```python
from build123d import *

# Parameters (mm, degrees)
BOSS_EXTRUDE2_DEPTH = 50.8
CUT_EXTRUDE2_START  = -10.16
SKETCH2_R           = 6.35
CUT_EXTRUDE2_DEPTH  = 19.997379


with BuildPart() as part:
    # Sketch1 → Boss-Extrude2 (new body)
    with BuildSketch(Plane.XY):
        with BuildLine():
            Line((-2.54, 7.184204897), (-2.54, 9.837377699))
            ThreePointArc((-2.54, 9.837377699), (-6.221703947, -8.032185257), (10.16, 0))
            ThreePointArc((10.16, 0), (8.032185257, 6.221703947), (2.54, 9.837377699))
            Line((2.54, 9.837377699), (2.54, 7.184204897))
            ThreePointArc((2.54, 7.184204897), (6.221703947, 4.399409051), (7.62, 0))
            ThreePointArc((7.62, 0), (-4.399409051, -6.221703947), (-2.54, 7.184204897))
        make_face()
    extrude(amount=BOSS_EXTRUDE2_DEPTH)

    # Sketch2 → Cut-Extrude2 (cut)
    with BuildSketch(Plane(origin=(0, 0, 0), x_dir=(1, 0, 0), z_dir=(0, 1, 0)).offset(CUT_EXTRUDE2_START)):
        with Locations(Location((0, -38.1, 0), (0, 0, 270))):  # turned: the seam where the file's is
            Circle(SKETCH2_R)
    extrude(amount=CUT_EXTRUDE2_DEPTH, mode=Mode.SUBTRACT)


solid = part.part
```
Here's how the part is built. I have some questions about the finished solid (model axes, mm). A direction names the side the tool comes from. Give positions to 0.01 mm unless a question says otherwise; leave off trailing zeros. Loops run counter-clockwise (first coordinate to the right, second up) from the corner with the lowest first, then second, coordinate; pieces in that order, holes last. Notation, with made-up numbers: (-38, 7) -> (11, 7) arc R8 cw to (11, 13) -> close; hole circle Ø10 at (12, 86). An arc over 180 degrees is marked (long way). Use one line per item in the form item = value. Start each with the question number.
1) Imagine slicing it at A-A (x = 0). Please give me the cut outline in (y, z), then the cut area to 3 significant figures.
2) Imagine slicing it at D-D (z = 23). Please give me the cut outline in (x, y), then the cut area to 3 significant figures.
3) Imagine slicing it at B-B (y = 5.25). Please give me the cut outline in (x, z).
4) Please list where these lines run through material, in increasing order: line 1 along X through (y, z) = (0, 41); line 2 along X through (y, z) = (4, 12.5); line 3 along Y through (x, z) = (0, 13.5).
5) For P1, Ø1, axis at x = 1, y = 7, coming from the -Z side; P2, Ø2, axis at y = 8, z = 21.5, coming from the -X side; P3, Ø0.8, axis at y = 8, z = 46.5, coming from the +X side; P4, Ø0.8, axis at y = 8.5, z = 13.5, coming from the +X side, each with a flat end and sliding along its axis, tell me the tip position at first contact or that it passes through.
6) Which directions (+Z, -Z, +X, -X, +Y, -Y) give clear straight access to the entire face, cutting with the end or side of a thin tool? Please do faces 5 (the face through (-2.54, 8, 47)), 6 (the face through (-6.35, 6.99, 38)), 7 (the face through (-8, -1, 0)).
7) Thinking about a two-plate mould opening in Z: for faces 1 (the face through (1.907, -7.89, 44.157)), 2 (the face through (-8, -1, 50.8)), 3 (the face through (6.35, 6.99, 38.2)), 4 (the face through (-2.54, 8, 16)), which applies, +Z half, -Z half, draft (parallel to the pull), parting line (faces both ways), or undercut?
8) Imagine slicing it at C-C (z = 38.1). Please give me the cut outline in (x, y).
Check values:
q1.outline = (-10.16, 0) -> (-7.62, 0) -> (-7.62, 31.75) -> (-10.16, 31.75) -> close; (-10.16, 44.45) -> (-7.62, 44.45) -> (-7.62, 50.8) -> (-10.16, 50.8) -> close
q1.area = 96.8 mm^2
q2.outline = (-2.54, 7.18) -> (-2.54, 9.84) arc R10.16 ccw (long way) to (2.54, 9.84) -> (2.54, 7.18) arc R7.62 cw (long way) to start
q2.area = 129 mm^2
q3.outline = (-8.7, 0) -> (-5.52, 0) -> (-5.52, 34.97) arc R6.35 cw to (-5.52, 41.23) -> (-5.52, 50.8) -> (-8.7, 50.8) -> close; (5.52, 0) -> (8.7, 0) -> (8.7, 50.8) -> (5.52, 50.8) -> (5.52, 41.23) arc R6.35 cw to (5.52, 34.97) -> close
q4.line_1 = -10.16 to -7.62, 7.62 to 10.16
q4.line_2 = -9.34 to -6.49, 6.49 to 9.34
q4.line_3 = -10.16 to -7.62
q5.P1 = through
q5.P2 = -7.36
q5.P3 = 6.74
q5.P4 = 6.13
q6.face_5 = +Z, -Z, +Y
q6.face_6 = +Y, -Y
q6.face_7 = -Z, +X, -X, +Y, -Y
q7.face_1 = undercut
q7.face_2 = +Z half
q7.face_3 = undercut
q7.face_4 = draft
q8.outline = (-6.35, -7.93) -> (-6.35, -4.21) arc R7.62 cw to (-6.35, 4.21) -> (-6.35, 7.93) arc R10.16 ccw to start; (6.35, -7.93) arc R10.16 ccw to (6.35, 7.93) -> (6.35, 4.21) arc R7.62 cw to (6.35, -4.21) -> close
